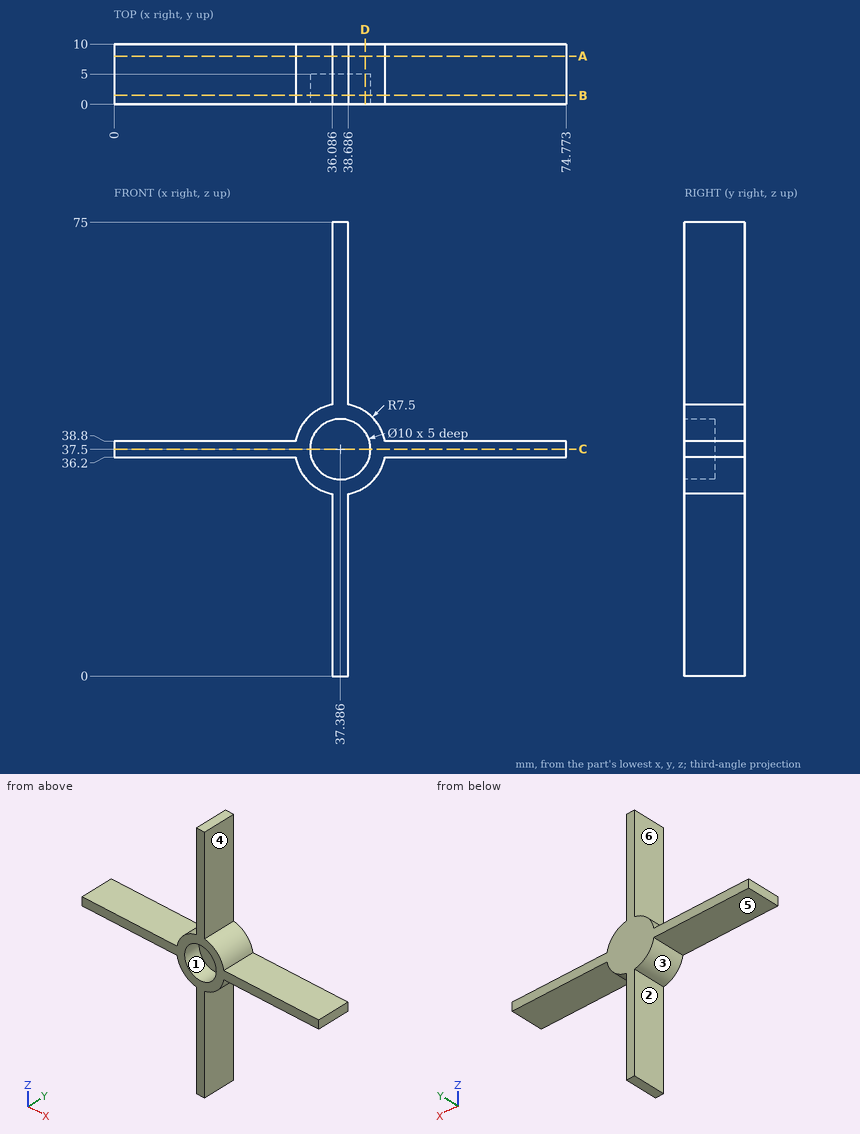
Job drawing, mm, ordinate dimensions from the low corner. One solid piece. A direction names the side the tool comes from. Coordinates: 2 decimals unless noted, no trailing zeros. Order: outer loops, then holes, each group sorted by start corner. A loop starts at its lowest first (then second) coordinate and runs counter-clockwise, first axis right, second up. Notation, with made-up numbers: (-5, 21.5) - (39, 21.5) arc R20 ccw to (39, 36.5) - close; hole circle Ø11 at (69, -39.5). An arc over 180 degrees is marked (long way). Write each question's results on one line, items separated by ' | '. Start each with the question number.
Item 1: Band-saw the part on D-D on x = 41.5. Write the cut outline in (y, z).
Item 2: Mould opens along Z. For the marked faces 1, 2 and 3 say: released by +Z, released by -Z, zero draft, split by the parting line, or undercut.
Item 3: Band-saw the part on A-A on y = 8. Write the cut outline in (x, z).
Item 4: Band-saw the part on B-B on y = 1.5. Write the cut outline in (x, z), and give its area (3 significant figures).
Item 5: Flat gauge pins, fed straight in: pin 1 (5 mm diameter, centred on y = 5.5, z = 63.5, fed in from -X); pin 2 (3 mm diameter, centred on x = 58, y = 5.5, fed in from -Z); pin 3 (11 mm diameter, centred on x = 35.5, z = 38, fed in from -Y); pin 4 (3 mm diameter, centred on y = 7.5, z = 7.5, fed in from +X). Where does each tip first touch, or does it go through?
Item 6: Band-saw the part on C-C on z = 37.5. Write the cut outline in (x, y).
Item 7: Tool access for the marked faces 4, 5 and 6: list every direction of +Z, -Z, +X, -X, +Y, -Y with a clear straight run to the whole face (end or side of a thin tool).
Item 8: Wall check: probe 1 along Z at (x, y) = (37, 2.5) (1 decimal); probe 2 along X at (y, z) = (1, 68); probe 3 along Z at (x, y) = (68, 8.25). Give the ranges that are in metal, low to high. Write a range as [from, to].
Numbers:
1) outline: (0, 31.23) - (10, 31.23) - (10, 43.77) - (0, 43.77) - (0, 40.34) - (5, 40.34) - (5, 34.66) - (0, 34.66) - close
2) face 1: undercut | face 2: zero draft | face 3: released by -Z
3) outline: (0, 36.2) - (30, 36.2) arc R7.5 ccw to (36.09, 30.11) - (36.09, 0) - (38.69, 0) - (38.69, 30.11) arc R7.5 ccw to (44.77, 36.2) - (74.77, 36.2) - (74.77, 38.8) - (44.77, 38.8) arc R7.5 ccw to (38.69, 44.89) - (38.69, 75) - (36.09, 75) - (36.09, 44.89) arc R7.5 ccw to (30, 38.8) - (0, 38.8) - close
4) outline: (0, 36.2) - (30, 36.2) arc R7.5 ccw to (36.09, 30.11) - (36.09, 0) - (38.69, 0) - (38.69, 30.11) arc R7.5 ccw to (44.77, 36.2) - (74.77, 36.2) - (74.77, 38.8) - (44.77, 38.8) arc R7.5 ccw to (38.69, 44.89) - (38.69, 75) - (36.09, 75) - (36.09, 44.89) arc R7.5 ccw to (30, 38.8) - (0, 38.8) - close; hole circle Ø10 at (37.39, 37.5) | area: 410 mm^2
5) pin 1: x = 36.09 | pin 2: z = 36.2 | pin 3: y = 0 | pin 4: x = 38.69
6) outline: (0, 0) - (32.39, 0) - (32.39, 5) - (42.39, 5) - (42.39, 0) - (74.77, 0) - (74.77, 10) - (0, 10) - close
7) face 4: +Z, +X, +Y, -Y | face 5: -Z, -X, +Y, -Y | face 6: +Z, -X, +Y, -Y
8) probe 1: [0, 32.5], [42.5, 75] | probe 2: [36.09, 38.69] | probe 3: [36.2, 38.8]
